Could you check a few things on this model? Use its own coordinates, in mm. Give positions to 0.01 mm unless a question says otherwise; leave off trailing zeros. Order: outer loops, then holes, each group sorted by start corner. A loop starts at its lowest first (then second) coordinate and runs counter-clockwise, first axis right, second up.
from build123d import *

# Parameters (mm, degrees)
BOSS_EXTRUDE1_DEPTH             = 6
LPATTERN1_COUNT                 = 5
LPATTERN1_PITCH                 = 2
SKETCH4_W                       = 10
SKETCH4_H                       = 6.004
BOSS_EXTRUDE3_DEPTH             = 6
M3X0_5_TAPPED_HOLE1_D           = 2.5
M3X0_5_TAPPED_HOLE1_CSINK_D     = 3.05
M3X0_5_TAPPED_HOLE1_CSINK_ANGLE = 90
FILLET1_R                       = 0.5
FILLET2_R                       = 0.15


with BuildPart() as part:
    # Sketch1 → Boss-Extrude1 (new, symmetric)
    with BuildSketch(Plane.XY):
        with BuildLine():
            Line((0, 0), (1, 0))
            Line((1, 0), (1, -1.004))
            ThreePointArc((1, -1.004), (0.705850588, -0.919639059), (0.501123596, -0.692202247))
            ThreePointArc((0.501123596, -0.692202247), (0.442388286, -0.542062154), (0.408543109, -0.384434783))
            ThreePointArc((0.408543109, -0.384434783), (0.358731646, -0.291228588), (0.259824575, -0.254))
            Line((0.259824575, -0.254), (0, -0.254))
            Line((0, -0.254), (0, 0))
        make_face()
    extrude(amount=BOSS_EXTRUDE1_DEPTH, both=True)

    # Mirror1: part across plane


with BuildPart() as part_1:
    add(part.part)
    add(part.part.mirror(Plane(origin=(1, 0, 6), x_dir=(0, 0, 1), z_dir=(-1, 0, 0))))


with BuildPart() as lpattern1_1:
    # LPattern1: pattern copy
    add(part_1.part.moved(Location(Vector(-1, 0, 0) * (1 * LPATTERN1_PITCH))))


with BuildPart() as lpattern1_2:
    # LPattern1: pattern copy
    add(part_1.part.moved(Location(Vector(-1, 0, 0) * (2 * LPATTERN1_PITCH))))


with BuildPart() as lpattern1_3:
    # LPattern1: pattern copy
    add(part_1.part.moved(Location(Vector(-1, 0, 0) * (3 * LPATTERN1_PITCH))))


with BuildPart() as lpattern1_4:
    # LPattern1: pattern copy
    add(part_1.part.moved(Location(Vector(-1, 0, 0) * (4 * LPATTERN1_PITCH))))


with BuildPart() as lpattern1_1_1:
    add(lpattern1_1.part)

    # Combine1: union LPattern1_4, part, LPattern1_3, LPattern1_2
    add(lpattern1_4.part)
    add(part_1.part)
    add(lpattern1_3.part)
    add(lpattern1_2.part)


with BuildPart() as body_2:
    # Sketch4 → Boss-Extrude3 (new, symmetric)
    with BuildSketch(Plane.XY):
        with Locations((-3, -3.002)):
            Rectangle(SKETCH4_W, SKETCH4_H)
    extrude(amount=BOSS_EXTRUDE3_DEPTH, both=True)

    # Combine2: cut LPattern1_1
    add(lpattern1_1_1.part, mode=Mode.SUBTRACT)

    # M3x0.5 Tapped Hole1 (through all)
    with Locations(Plane.ZY.offset(8)):
        with Locations((0, -3.504)):
            CounterSinkHole(M3X0_5_TAPPED_HOLE1_D / 2, M3X0_5_TAPPED_HOLE1_CSINK_D / 2, counter_sink_angle=M3X0_5_TAPPED_HOLE1_CSINK_ANGLE)

    # Fillet1
    fillet1_edges = [body_2.edges().sort_by_distance(p)[0] for p in [
        (2, -6.004, 0),
        (-8, -6.004, 0),
    ]]
    fillet(fillet1_edges, radius=FILLET1_R)

    # Fillet2
    fillet2_edges = [body_2.edges().sort_by_distance(p)[0] for p in [
        (-8, -0.254, 0),
        (2, -0.254, 0),
    ]]
    fillet(fillet2_edges, radius=FILLET2_R)


solid = body_2.part
Item 1: Please list where these lines run through material, in increasing order: line 1 along Y through (x, z) = (-3.5, 0.75); line 2 along Y through (x, z) = (-6, 0); line 3 along X through (y, z) = (-0.7, 2.5) (3 decimals).
Findings:
line 1: y = -6 to -4.5, -2.5 to -0.69
line 2: y = -6 to -4.75, -2.25 to -0.25
line 3: x = -8 to -7.495, -6.505 to -5.495, -4.505 to -3.495, -2.505 to -1.495, -0.505 to 0.505, 1.495 to 2
Item 2: We'd pull the mould along Z, two halves only. Please class faces 1 (the flat face through (-3, -3, 6)), 2 (the flat face through (2, -2, 0)), 3 (the cylindrical face through (-2.794, -2.265, 0.163)): +Z half, -Z half, draft (parallel to the pull), parting line (faces both ways), or undercut.
Findings:
face 1: +Z half
face 2: draft
face 3: undercut
Item 3: Imagine slicing it at A-A on x = -5.25. List the corners of the cut face in (y, z) for me.
Findings:
outline: (-6, -6) - (-0.94, -6) - (-0.94, 6) - (-6, 6) - close; hole circle Ø2.5 at (-3.5, 0)
